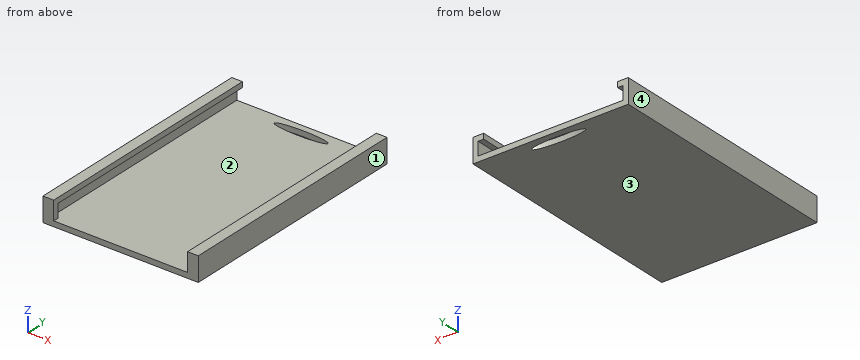
```python
from build123d import *

# Parameters (mm, degrees)
F0_W     = 58
F0_H     = 90
F1_DEPTH = 9
F2_W     = 50
F2_H     = 90
F3_DEPTH = 7
F4_W     = 54.2
F4_H     = 5
F5_DEPTH = 88
F7_DEPTH = 25


# Not quite as in the source:
# - a feature names something its author has since deleted; it is built from what else it names


with BuildPart() as f1:
    # F0 (on Top) → F1 (new body)
    with BuildSketch(Plane.XY):
        Rectangle(F0_W, F0_H)
    extrude(amount=F1_DEPTH)

    # F2 (on face) → F3 (cut)
    with BuildSketch(Plane.XY.offset(9)):
        Rectangle(F2_W, F2_H)
    extrude(amount=-F3_DEPTH, mode=Mode.SUBTRACT)

    # F4 (on face) → F5 (cut)
    with BuildSketch(Plane(origin=(0, 45, 0), x_dir=(-1, 0, 0), z_dir=(0, 1, 0))):
        with Locations((0, 4.5)):
            Rectangle(F4_W, F4_H)
    extrude(amount=-F5_DEPTH, mode=Mode.SUBTRACT)

    # F6 (on face) → F7 (cut)
    with BuildSketch(Plane.XY.offset(2)):
        with BuildLine():
            add(Edge.make_bspline(
                [(10.0087067112, 41.0774275661), (10.0087067112, 43.8166453426), (-5.0043533556, 42.4470364543), (-20.0174134225, 41.0774275661), (-5.0043533556, 39.7078186778), (10.0087067112, 38.3382097895), (10.0087067112, 41.0774275661)],
                knots=[0, 0, 0, 2.0943951024, 2.0943951024, 4.1887902048, 4.1887902048, 6.2831853072, 6.2831853072, 6.2831853072], degree=2, weights=[1, 0.5, 1, 0.5, 1, 0.5, 1]))
        make_face()
    extrude(amount=-F7_DEPTH, mode=Mode.SUBTRACT)


solid = f1.part
```
Verification items for the finished model (mm, model axes). Face numbers are marked on the shaded views. Round coordinates to 2 decimals unless told otherwise and drop trailing zeros. Loops run counter-clockwise (first coordinate to the right, second up) from the corner with the lowest first, then second, coordinate; pieces in that order, holes last. Notation, with made-up numbers: (49, 43) -> (88, 43) arc R6 ccw to (88, 53) -> close; hole circle Ø9 at (10, 55). An arc over 180 degrees is marked (long way). Answer as a JSON object with one key per item and string values.
Q1. Scan lines: line 1 (X direction, y = -25.5, z = 5.75); line 2 (X direction, y = -9, z = 8.25); line 3 (Y direction, x = -26, z = 4.75). Record each from-to range of solid material in increasing order. Write a range as from..to.
Data:
{"line 1": "x = -29..-27.1, 27.1..29", "line 2": "x = -29..-25, 25..29", "line 3": "y = -45..-43"}
Q2. Section check C-C (x = -12.5). Record the boundary of the cut face in (y, z).
Data:
{"outline": "(-45, 0) -> (45, 0) -> (45, 2) -> (-45, 2) -> close"}
Q3. Section check B-B (y = -2). Record the boundary of the cut face in (x, z).
Data:
{"outline": "(-29, 0) -> (29, 0) -> (29, 9) -> (25, 9) -> (25, 7) -> (27.1, 7) -> (27.1, 2) -> (-27.1, 2) -> (-27.1, 7) -> (-25, 7) -> (-25, 9) -> (-29, 9) -> close"}
Q4. Section check A-A (z = 5.25). Record the boundary of the cut face in (x, y), then the cut area to 3 significant figures.
Data:
{"outline": "(-29, -45) -> (-25, -45) -> (-25, -43) -> (-27.1, -43) -> (-27.1, 45) -> (-29, 45) -> close; (25, -45) -> (29, -45) -> (29, 45) -> (27.1, 45) -> (27.1, -43) -> (25, -43) -> close", "area": "350 mm2"}
Q5. Go/stop test with flat-tipped pins: P1, Ø2.5, axis at x = 26.5, z = 5.5, coming from the +Y side; P2, Ø8, axis at x = 14.5, y = 35, coming from the +Z side. Record where each tip stops, or that it passes through.
Data:
{"P1": "stops at y = 45", "P2": "stops at z = 2"}
Q6. Draft check along X on the marked faces 1, 2, 3 and 4. Enter one of: pulls with the +X half, pulls with the -X half, needs draft (parallel to the pull), parting line crosses it, or undercut.
Data:
{"face 1": "pulls with the +X half", "face 2": "undercut", "face 3": "needs draft", "face 4": "pulls with the -X half"}
